Read the model definition and answer for the solid it produces. Units are mm, in the model's axes. Face numbers are marked on the shaded views. A direction names the side the tool comes from. Coordinates: 2 decimals unless noted, no trailing zeros. Order: outer loops, then holes, each group sorted by start corner. A loop starts at its lowest first (then second) coordinate and runs counter-clockwise, first axis right, second up.
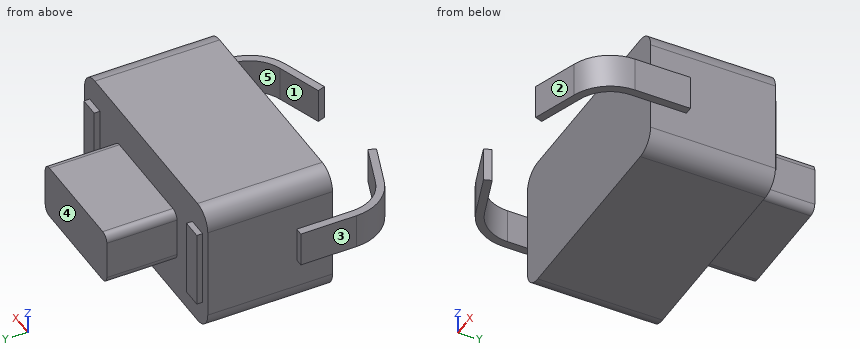
```python
from build123d import *

# Parameters (mm, degrees)
SKETCH1_W           = 6
SKETCH1_H           = 3.4
BOSS_EXTRUDE1_DEPTH = 3.2
SKETCH2_W           = 3
SKETCH2_H           = 1.4
BOSS_EXTRUDE2_DEPTH = 1.8
SKETCH2_3_W         = 0.5
SKETCH2_3_H         = 2
BOSS_EXTRUDE3_DEPTH = 0.15
FILLET1_R           = 0.2
FILLET3_R           = 0.5
SKETCH3_W           = 0.2
SKETCH3_H           = 0.9


with BuildPart() as part:
    # Sketch1 → Boss-Extrude1 (new body)
    with BuildSketch(Plane(origin=(0, 0, 0), x_dir=(1, 0, 0), z_dir=(0, 1, 0))):
        Rectangle(SKETCH1_W, SKETCH1_H)
    extrude(amount=BOSS_EXTRUDE1_DEPTH)

    # Sketch2 → Boss-Extrude2 (add)
    with BuildSketch(Plane(origin=(0, 3.2, 0), x_dir=(1, 0, 0), z_dir=(0, 1, 0))):
        Rectangle(SKETCH2_W, SKETCH2_H)
    extrude(amount=BOSS_EXTRUDE2_DEPTH)

    # Sketch2<3> → Boss-Extrude3 (add)
    with BuildSketch(Plane(origin=(0, 3.2, 0), x_dir=(1, 0, 0), z_dir=(0, 1, 0))):
        with Locations((-2.5, 0)):
            Rectangle(SKETCH2_3_W, SKETCH2_3_H)
        with Locations((2.5, 0)):
            Rectangle(SKETCH2_3_W, SKETCH2_3_H)
    extrude(amount=BOSS_EXTRUDE3_DEPTH)

    # Fillet1
    fillet1_edges = [part.edges().sort_by_distance(p)[0] for p in [
        (-1.5, 4.1, -0.7),
        (-1.5, 4.1, 0.7),
        (1.5, 4.1, 0.7),
        (1.5, 4.1, -0.7),
    ]]
    fillet(fillet1_edges, radius=FILLET1_R)

    # Fillet3
    fillet3_edges = [part.edges().sort_by_distance(p)[0] for p in [
        (-3, 1.6, -1.7),
        (3, 1.6, -1.7),
        (3, 1.6, 1.7),
        (-3, 1.6, 1.7),
    ]]
    fillet(fillet3_edges, radius=FILLET3_R)

    # Sweep1: sweep along a path in Sketch4
    with BuildLine(Plane.XY) as sweep1_path:
        Line((-1.204114161, -1.850245601), (-2.331506907, -1.454106562))
        ThreePointArc((-2.331506907, -1.454106562), (-2.815937163, -1.088794364), (-3, -0.51065377))
        Line((-3, -0.51065377), (-3, 0))
        Line((-3, 0), (-3, 0.917319166))
    # Sketch3 → Sweep1 (sweep)
    with BuildSketch(Plane.XZ):
        with Locations((-3.1, 0)):
            Rectangle(SKETCH3_W, SKETCH3_H)
    sweep1 = sweep(path=sweep1_path.line)

    # Mirror1: Sweep1 across plane
    add(sweep1.mirror(Plane(origin=(0, 0, 0), x_dir=(0, 0, 1), z_dir=(1, 0, 0))))


solid = part.part
```
1) Determine the mould class of the marked faces 1, 2 and 3 for opening direction Y: pulls with the +Y half, pulls with the -Y half, needs draft (parallel to the pull), parting line crosses it, or undercut.
A:
face 1: undercut
face 2: pulls with the -Y half
face 3: needs draft
2) A cutting plane is placed at A-A, the plane x = -1.75. Determine the outline of the cut face in (y, z).
A:
outline: (-1.87, -0.45) - (-1.66, -0.45) - (-1.66, 0.45) - (-1.87, 0.45) - close; (0, -1.7) - (3.2, -1.7) - (3.2, 1.7) - (0, 1.7) - close
3) Which of the six approach directions +Z, -Z, +X, -X, +Y, -Y give full straight-line access (tool end or side, diameter ignored) to the marked faces 4 and 5?
A:
face 4: +Z, -Z, +X, -X, +Y
face 5: +Z, -Z
4) Flat-ended cylindrical pins translate along their axes: pin 1 Ø1.4 at (x, y) = (0, 4.5) entering from +Z; pin 2 Ø1.6 at (x, y) = (2.5, -1) entering from -Z; pin 3 Ø1.6 at (x, y) = (2.5, -1) entering from +Z. Find the tip coordinate at first contact, or state that the pin passes through.
A:
pin 1: stops at z = 0.7
pin 2: stops at z = -0.45
pin 3: stops at z = 0.45
5) Straight lines are drawn through the part: line 1 (Y direction, x = -1, z = 0.65); line 2 (Y direction, x = 2.75, z = 1.45); line 3 (X direction, y = 2.25, z = 0.35). For each, find the intervals that lie inside material, in ascending order.
A:
line 1: y = 0 to 5
line 2: y = 0 to 3.2
line 3: x = -3 to 3
6) A cutting plane is placed at C-C, the plane y = 1.5. Determine the outline of the cut face in (x, z).
A:
outline: (-3, -1.2) arc R0.5 ccw to (-2.5, -1.7) - (2.5, -1.7) arc R0.5 ccw to (3, -1.2) - (3, 1.2) arc R0.5 ccw to (2.5, 1.7) - (-2.5, 1.7) arc R0.5 ccw to (-3, 1.2) - close
7) A cutting plane is placed at B-B, the plane x = 0. Determine the outline of the cut face in (y, z).
A:
outline: (0, -1.7) - (3.2, -1.7) - (3.2, -0.7) - (5, -0.7) - (5, 0.7) - (3.2, 0.7) - (3.2, 1.7) - (0, 1.7) - close
